Source: CAD feature listing. Evaluate the final solid. Frame: model axes, mm. A direction names the side the tool comes from. Give positions to 0.01 mm unless a question says otherwise; leave off trailing zeros. Write each loop counter-clockwise with the first axis right and the second up, starting at its lowest first coordinate (ties: lowest second). Pieces come first, ordered by that corner, then holes.
```python
from build123d import *

# Parameters (mm, degrees)
SKETCH1_W               = 63.5
SKETCH1_H               = 190.5
BOSS_EXTRUDE1_DEPTH     = 3.175
SKETCH3_R               = 2.0828
CUT_EXTRUDE2_DEPTH      = 526.850378691
SKETCH4_R               = 2.0828
CUT_EXTRUDE4_DEPTH      = 526.850378691
FILLET2_R               = 3.175
CUT_EXTRUDE5_DEPTH      = 526.850378691
CUT_EXTRUDE5_DEPTH_BACK = 526.850378691
SKETCH5_W               = 142.875
SKETCH5_H               = 355.6


with BuildPart() as part:
    # Sketch1 → Boss-Extrude1 (new body)
    with BuildSketch(Plane(origin=(0, 0, 0), x_dir=(1, 0, 0), z_dir=(0, 1, 0))):
        Polygon((-242.686835374, -133.432512515), (-242.686835374, -385.491221995), (-242.686835374, -387.371651362), (-191.886835374, -438.171651362), (239.913164626, -438.171651362), (290.713164626, -387.371651362), (290.713164626, -133.371651362), (176.413164626, -82.571651362), (176.413164626, -133.371651362), (74.813164626, -196.871651362), (-26.786835374, -196.871651362), (-128.386835374, -133.371651362), (-128.386835374, -82.571651362), (-242.686835374, -133.371651362), align=None)
        with Locations((233.563164626, -243.80020948)):
            Rectangle(SKETCH1_W, SKETCH1_H, mode=Mode.SUBTRACT)
        with Locations((-185.536835374, -243.80020948)):
            Rectangle(SKETCH1_W, SKETCH1_H, mode=Mode.SUBTRACT)
    extrude(amount=BOSS_EXTRUDE1_DEPTH)

    # Sketch3 → Cut-Extrude2 (cut, through all)
    with BuildSketch(Plane(origin=(0, 0, 0), x_dir=(1, 0, 0), z_dir=(0, 1, 0))):
        with Locations(Location((-114.278235374, -270.125471314, 0), (0, 0, 270))):
            Circle(SKETCH3_R)
        with Locations(Location((-143.449035374, -284.13540948, 0), (0, 0, 270))):
            Circle(SKETCH3_R)
        with Locations(Location((-114.278235374, -217.474947647, 0), (0, 0, 270))):
            Circle(SKETCH3_R)
        with Locations(Location((-143.449035374, -203.46500948, 0), (0, 0, 270))):
            Circle(SKETCH3_R)
        with Locations(Location((191.475364626, -284.13540948, 0), (0, 0, 270))):
            Circle(SKETCH3_R)
        with Locations(Location((162.304564626, -270.125471314, 0), (0, 0, 270))):
            Circle(SKETCH3_R)
        with Locations(Location((162.304564626, -217.474947647, 0), (0, 0, 270))):
            Circle(SKETCH3_R)
        with Locations(Location((191.475364626, -203.46500948, 0), (0, 0, 270))):
            Circle(SKETCH3_R)
    extrude(amount=CUT_EXTRUDE2_DEPTH, mode=Mode.SUBTRACT)

    # Sketch4 → Cut-Extrude4 (cut, through all)
    with BuildSketch(Plane(origin=(0, 0, 0), x_dir=(1, 0, 0), z_dir=(0, 1, 0))):
        with Locations(Location((111.325664626, -210.298576853, 0), (0, 0, 270))):
            Circle(SKETCH4_R)
        with Locations(Location((111.325664626, -413.498576853, 0), (0, 0, 270))):
            Circle(SKETCH4_R)
        with Locations(Location((-63.299335374, -413.498576853, 0), (0, 0, 90))):
            Circle(SKETCH4_R)
        with Locations(Location((-63.299335374, -210.298576853, 0), (0, 0, 90))):
            Circle(SKETCH4_R)
        with BuildLine():
            Line((-50.599335374, -216.648576853), (98.625664626, -216.648576853))
            Line((98.625664626, -216.648576853), (98.625664626, -232.523576853))
            ThreePointArc((98.625664626, -232.523576853), (108.150664626, -242.048576853), (98.625664626, -251.573576853))
            Line((98.625664626, -251.573576853), (98.625664626, -384.923576853))
            ThreePointArc((98.625664626, -384.923576853), (108.150664626, -394.448576853), (98.625664626, -403.973576853))
            Line((98.625664626, -403.973576853), (98.625664626, -419.848576853))
            Line((98.625664626, -419.848576853), (-50.599335374, -419.848576853))
            Line((-50.599335374, -419.848576853), (-50.599335374, -403.973576853))
            ThreePointArc((-50.599335374, -403.973576853), (-60.124335374, -394.448576853), (-50.599335374, -384.923576853))
            Line((-50.599335374, -384.923576853), (-50.599335374, -251.573576853))
            ThreePointArc((-50.599335374, -251.573576853), (-60.124335374, -242.048576853), (-50.599335374, -232.523576853))
            Line((-50.599335374, -232.523576853), (-50.599335374, -216.648576853))
        make_face()
    extrude(amount=CUT_EXTRUDE4_DEPTH, mode=Mode.SUBTRACT)

    # Fillet2
    fillet2_edges = [part.edges().sort_by_distance(p)[0] for p in [
        (98.625664626, 1.5875, 419.848576853),
        (98.625664626, 1.5875, 216.648576853),
        (-50.599335374, 1.5875, 216.648576853),
        (-50.599335374, 1.5875, 419.848576853),
    ]]
    fillet(fillet2_edges, radius=FILLET2_R)

    # Sketch5 → Cut-Extrude5 (cut, two sides: drawn at the far end of the back side and taken through both)
    with BuildSketch(Plane(origin=(0, 3.175, 0), x_dir=(1, 0, 0), z_dir=(0, 1, 0)).offset(-CUT_EXTRUDE5_DEPTH_BACK)):
        with Locations((-171.249335374, -260.371651362)):
            Rectangle(SKETCH5_W, SKETCH5_H)
        with Locations((219.275664626, -260.371651362)):
            Rectangle(SKETCH5_W, SKETCH5_H)
    extrude(amount=CUT_EXTRUDE5_DEPTH + CUT_EXTRUDE5_DEPTH_BACK, mode=Mode.SUBTRACT)


solid = part.part
```
1. Line query: probe 1 along Z at (x, y) = (9.5, 0.8); probe 2 along X at (y, z) = (2.4, 414); probe 3 along X at (y, z) = (2.45, 325). Output: solid intervals per line, ascending.
2. Section query A-A (x = 26). Return loops of the section in (y, z) (3 decimals).
3. Pull-direction query (X, two-part tool) for faces 4 (the cylindrical face through (-60.12, 1.57, 242.26)), 5 (the flat face through (-60, 3.175, 293)); classes: pulls with the +X half, pulls with the -X half, needs draft (parallel to the pull), parting line crosses it, or undercut.
4. Pin query (flat end, axial travel): P1, Ø3.5, axis at x = -63.3, z = 413.5, coming from the +Y side; P2, Ø1.6, axis at x = -11.5, y = 1, coming from the -Z side; P3, Ø1, axis at x = 99.5, y = 2.5, coming from the -Z side. Return the tip coordinate at first contact, or that it passes through.
5. Section query B-B (z = 284.5). Return loops of the section in (x, y) (3 decimals), plus the area to 4 significant figures.
6. Access query for faces 1 (the cylindrical face through (-60.12, 1.57, 394.66)), 2 (the flat face through (-60, 0, 293)), 3 (the flat face through (-62.79, 1.57, 174.37)). Directions: +Z, -Z, +X, -X, +Y, -Y. A direction counts if a zero-diameter tool reaches every point of the face in a straight line with its end or side. Return the directions, or none.
7. Section query D-D (x = -54). Return loops of the section in (y, z) (3 decimals), plus the area to 3 significant figures.
8. Section query C-C (y = 2.15). Return loops of the section in (x, z) (3 decimals).
The answers:
1. probe 1: z = 196.87 to 216.65, 419.85 to 438.17
1. probe 2: x = -99.81 to -65.32, -61.28 to -50.6, 98.63 to 109.3, 113.35 to 147.84
1. probe 3: x = -99.81 to -50.6, 98.63 to 147.84
2. outline: (0, 196.872) - (3.175, 196.872) - (3.175, 216.649) - (0, 216.649) - close; (0, 419.849) - (3.175, 419.849) - (3.175, 438.172) - (0, 438.172) - close
3. face 4: undercut
3. face 5: needs draft
4. P1: passes through
4. P2: stops at z = 196.87
4. P3: stops at z = 181.13
5. outline: (-99.812, 0) - (-50.599, 0) - (-50.599, 3.175) - (-99.812, 3.175) - close; (98.626, 0) - (147.838, 0) - (147.838, 3.175) - (98.626, 3.175) - close
5. area: 312.5 mm2
6. face 1: +Y, -Y
6. face 2: +Z, -Z, +X, -X, -Y
6. face 3: -Z, +Y, -Y
7. outline: (0, 179.863) - (3.175, 179.863) - (3.175, 233.151) - (0, 233.151) - close; (0, 250.946) - (3.175, 250.946) - (3.175, 385.551) - (0, 385.551) - close; (0, 403.346) - (3.175, 403.346) - (3.175, 438.172) - (0, 438.172) - close
7. area: 707 mm2
8. outline: (-99.812, 151.231) - (-26.787, 196.872) - (74.813, 196.872) - (147.838, 151.231) - (147.838, 438.172) - (-99.812, 438.172) - close; hole circle Ø4.166 at (-63.299, 210.299); hole circle Ø4.166 at (-63.299, 413.499); hole (-50.599, 219.824) arc R3.175 ccw to (-47.424, 216.649) - (95.451, 216.649) arc R3.175 ccw to (98.626, 219.824) - (98.626, 232.524) arc R9.525 ccw to (98.626, 251.574) - (98.626, 384.924) arc R9.525 ccw to (98.626, 403.974) - (98.626, 416.674) arc R3.175 ccw to (95.451, 419.849) - (-47.424, 419.849) arc R3.175 ccw to (-50.599, 416.674) - (-50.599, 403.974) arc R9.525 ccw to (-50.599, 384.924) - (-50.599, 251.574) arc R9.525 ccw to (-50.599, 232.524) - close; hole circle Ø4.166 at (111.326, 210.299); hole circle Ø4.166 at (111.326, 413.499)
